from build123d import *

# Parameters (mm, degrees)
SKETCH_1_W                = 105
SKETCH_1_H                = 10
EXTRUDE_3_DEPTH           = 10
EXTRUDE_3_DEPTH_BACK      = 20
SKETCH_11_R               = 105
SKETCH_11_R_2             = 100
EXTRUDE_START             = 20
SKETCH_12_R               = 105
SKETCH_12_R_2             = 100
EXTRUDE_4_DEPTH           = 20
SKETCH_4_R                = 25.5
SKETCH_4_R_2              = 20.5
EXTRUDE_6_DEPTH           = 20
EXTRUDE_START_2           = -31.598350223
EXTRUDE_7_OUTLINE_R       = 26
EXTRUDE_7_OUTLINE_R_2     = 21
EXTRUDE_7_DEPTH           = 30.598350223
SKETCH_6_R                = 20
CUT_EXTRUDE_1_DEPTH       = 174.040821302
CUT_EXTRUDE_8_DEPTH       = 10
CUT_EXTRUDE_START         = -4.05
SKETCH_17_W               = 12.2
SKETCH_17_H               = 22.6
CUT_EXTRUDE_9_DEPTH       = 6.15
CUT_EXTRUDE_START_2       = -35
CUT_EXTRUDE_10_DEPTH      = 35.9
SKETCH_21_W               = 12.48598734
SKETCH_21_H               = 3.935393954
CUT_EXTRUDE_11_DEPTH      = 174.040821302
SKETCH_23_W               = 21.5
SKETCH_23_H               = 4
MIRROR_START              = -126.5
MIRROR_3_OUTLINE_R        = 26
MIRROR_3_OUTLINE_R_2      = 24
MIRROR_3_DEPTH            = 21.5
SKETCH_24_R               = 20
CUT_EXTRUDE_12_DEPTH      = 174.040821302
SKETCH_25_W               = 5.25
SKETCH_25_H               = 10
CUT_EXTRUDE_13_DEPTH      = 1
EXTRUDE_8_DEPTH           = 35
FILLET_1_R                = 10
FILLET_1_OF_MIRROR_4_R    = 10
M5X0_8_1_D                = 4.2
SKETCH_38_R               = 2.55
CUT_EXTRUDE_17_DEPTH      = 190.567335177
M5X0_8_2_D                = 4.2
CUT_EXTRUDE_18_DEPTH      = 183.219119633
CUT_EXTRUDE_18_DEPTH_BACK = 183.219119633
SKETCH_39_R               = 2.55
CUT_EXTRUDE_14_DEPTH      = 183.219119633
CUT_EXTRUDE_14_DEPTH_BACK = 183.219119633
SKETCH_34_W               = 208.658629851
SKETCH_34_H               = 276.195432186


with BuildPart() as part:
    # 草图1 → 旋转1 (revolve)
    with BuildSketch(Plane(origin=(0, 0, 0), x_dir=(1, 0, 0), z_dir=(0, 1, 0))):
        with Locations((52.5, 5)):
            Rectangle(SKETCH_1_W, SKETCH_1_H)
    revolve(axis=Axis((0, 0, 0), (0, 0, -1)))

    # 草图11 → 凸台-拉伸3 (add, two sides: drawn at the far end of the back side and taken through both)
    with BuildSketch(Plane.XY.offset(-EXTRUDE_3_DEPTH_BACK)):
        Circle(SKETCH_11_R)
        Circle(SKETCH_11_R_2, mode=Mode.SUBTRACT)
    extrude(amount=EXTRUDE_3_DEPTH + EXTRUDE_3_DEPTH_BACK)

    # 草图12 → 凸台-拉伸4 (add)
    with BuildSketch(Plane.XY.offset(10).offset(EXTRUDE_START)):
        Circle(SKETCH_12_R)
        Circle(SKETCH_12_R_2, mode=Mode.SUBTRACT)
    extrude_4 = extrude(amount=-EXTRUDE_4_DEPTH)

    # 镜向1: 凸台-拉伸4 across plane
    add(extrude_4.mirror(Plane.XY.offset(-5)))

    # 草图4 → 凸台-拉伸6 (add)
    with BuildSketch(Plane(origin=(100, 0, 0), x_dir=(0, 0, -1), z_dir=(1, 0, 0))):
        with Locations((5, 0)):
            Circle(SKETCH_4_R)
        with Locations((5, 0)):
            Circle(SKETCH_4_R_2, mode=Mode.SUBTRACT)
    extrude(amount=EXTRUDE_6_DEPTH)

    # 凸台-拉伸7: read off the stored shape, not the designer's step
    # 凸台-拉伸7 outline → 凸台-拉伸7 (add)
    with BuildSketch(Plane(origin=(-100, 0, 0), x_dir=(0, 0, -1), z_dir=(1, 0, 0)).offset(EXTRUDE_START_2)):
        with Locations((5, 0)):
            Circle(EXTRUDE_7_OUTLINE_R)
        with Locations((5, 0)):
            Circle(EXTRUDE_7_OUTLINE_R_2, mode=Mode.SUBTRACT)
    extrude(amount=EXTRUDE_7_DEPTH)

    # 草图6 → 切除-拉伸1 (cut, through all)
    with BuildSketch(Plane.XY):
        with Locations((0, -70)):
            Circle(SKETCH_6_R)
        with Locations(Location((0, 70, 0), (0, 0, 180))):
            Circle(SKETCH_6_R)
    extrude(amount=-CUT_EXTRUDE_1_DEPTH, mode=Mode.SUBTRACT)

    # 草图16 → 切除-拉伸8 (cut)
    with BuildSketch(Plane(origin=(105, 0, 0), x_dir=(0, 0, -1), z_dir=(1, 0, 0))):
        with BuildLine():
            ThreePointArc((7.301532566, -5.323809524), (5, 5.8), (2.698467434, -5.323809524))
            ThreePointArc((2.698467434, -5.323809524), (5, -8.8), (7.301532566, -5.323809524))
        make_face()
    cut_extrude_8 = extrude(amount=-CUT_EXTRUDE_8_DEPTH, mode=Mode.SUBTRACT)

    # 草图17 → 切除-拉伸9 (cut)
    with BuildSketch(Plane(origin=(100, 0, 0), x_dir=(0, 0, -1), z_dir=(1, 0, 0)).offset(CUT_EXTRUDE_START)):
        with Locations((4.890474786, -5.5)):
            Rectangle(SKETCH_17_W, SKETCH_17_H)
    cut_extrude_9 = extrude(amount=CUT_EXTRUDE_9_DEPTH, mode=Mode.SUBTRACT)

    # 草图19 → 切除-拉伸10 (cut)
    with BuildSketch(Plane(origin=(95.95, 0, 0), x_dir=(0, 0, -1), z_dir=(1, 0, 0)).offset(CUT_EXTRUDE_START_2)):
        Polygon((-1.122566441, -16.8), (-1.122566441, 5.8), (-1.122566441, 10.8), (11.077433559, 10.8), (11.077433559, 5.8), (11.077433559, -16.8), (11.077433559, -21.6), (-1.122566441, -21.6), align=None)
    cut_extrude_10 = extrude(amount=CUT_EXTRUDE_10_DEPTH, mode=Mode.SUBTRACT)

    # 镜向2: 切除-拉伸8, 切除-拉伸9, 切除-拉伸10 across plane
    add(cut_extrude_8.mirror(Plane(origin=(0, 0, 0), x_dir=(0, 0, 1), z_dir=(1, 0, 0))), mode=Mode.SUBTRACT)
    add(cut_extrude_9.mirror(Plane(origin=(0, 0, 0), x_dir=(0, 0, 1), z_dir=(1, 0, 0))), mode=Mode.SUBTRACT)
    add(cut_extrude_10.mirror(Plane(origin=(0, 0, 0), x_dir=(0, 0, 1), z_dir=(1, 0, 0))), mode=Mode.SUBTRACT)

    # 草图21 → 切除-拉伸11 (cut, through all)
    with BuildSketch(Plane.XY):
        with Locations((-80.471231892, 15.58208287)):
            Rectangle(SKETCH_21_W, SKETCH_21_H)
        with Locations((-80.471231892, -26.38208287)):
            Rectangle(SKETCH_21_W, SKETCH_21_H)
        with Locations((80.471231892, -26.38208287)):
            Rectangle(SKETCH_21_W, SKETCH_21_H)
        with Locations((80.471231892, 15.58208287)):
            Rectangle(SKETCH_21_W, SKETCH_21_H)
    extrude(amount=-CUT_EXTRUDE_11_DEPTH, mode=Mode.SUBTRACT)

    # 草图23 → 切除-旋转1 (revolve, cut)
    with BuildSketch(Plane.XY.offset(-5), mode=Mode.PRIVATE) as cut_revolve_1_sk:
        with Locations((115.75, 26)):
            Rectangle(SKETCH_23_W, SKETCH_23_H)
    revolve(cut_revolve_1_sk.sketch.rotate(Axis((120, 0, -5), (-1, 0, 0)), 90), axis=Axis((120, 0, -5), (-1, 0, 0)), mode=Mode.SUBTRACT)

    # 镜向3: read off the stored shape, not the designer's step
    # 镜向3 outline → 镜向3 (cut)
    with BuildSketch(Plane.YZ.offset(MIRROR_START)):
        with Locations((0, -5)):
            Circle(MIRROR_3_OUTLINE_R)
        with Locations((0, -5)):
            Circle(MIRROR_3_OUTLINE_R_2, mode=Mode.SUBTRACT)
    extrude(amount=MIRROR_3_DEPTH, mode=Mode.SUBTRACT)

    # 草图24 → 切除-拉伸12 (cut, through all)
    with BuildSketch(Plane.XY):
        Circle(SKETCH_24_R)
        with BuildLine():
            Line((-86.979425588, 23.120975852), (-48.321903105, 12.844986584))
            ThreePointArc((-48.321903105, 12.844986584), (0, 50), (48.321903105, 12.844986584))
            Line((48.321903105, 12.844986584), (86.979425588, 23.120975852))
            ThreePointArc((86.979425588, 23.120975852), (0, 90), (-86.979425588, 23.120975852))
        make_face()
        with BuildLine():
            Line((46.279615655, -18.926097718), (83.303308179, -34.066975893))
            ThreePointArc((83.303308179, -34.066975893), (0, -90), (-83.303308179, -34.066975893))
            Line((-83.303308179, -34.066975893), (-46.279615655, -18.926097718))
            ThreePointArc((-46.279615655, -18.926097718), (0, -50), (46.279615655, -18.926097718))
        make_face()
    extrude(amount=-CUT_EXTRUDE_12_DEPTH, mode=Mode.SUBTRACT)

    # 草图25 → 切除-拉伸13 (cut)
    with BuildSketch(Plane.XZ.offset(-5.8)):
        with Locations((99.475, -5)):
            Rectangle(SKETCH_25_W, SKETCH_25_H)
    extrude(amount=-CUT_EXTRUDE_13_DEPTH, mode=Mode.SUBTRACT)

    # 草图26 → 凸台-拉伸8 (add, symmetric)
    with BuildSketch(Plane.XY.offset(-5)):
        with BuildLine():
            Line((-10, 104.522724802), (-10, 119.522724802))
            Line((-10, 119.522724802), (10, 119.522724802))
            Line((10, 119.522724802), (10, 104.522724802))
            ThreePointArc((10, 104.522724802), (0, 105), (-10, 104.522724802))
        make_face()
    extrude_8 = extrude(amount=EXTRUDE_8_DEPTH, both=True)

    # 圆角1
    fillet_1_edges = [part.edges().sort_by_distance(p)[0] for p in [
        (0, 119.522724802, -40),
        (0, 119.522724802, 30),
    ]]
    fillet(fillet_1_edges, radius=FILLET_1_R)

    # 镜向4: 凸台-拉伸8 across plane
    add(extrude_8.mirror(Plane.ZX))

    # 圆角1 of 镜向4
    fillet_1_of_mirror_4_edges = [part.edges().sort_by_distance(p)[0] for p in [
        (0, -119.522724802, -40),
        (0, -119.522724802, 30),
    ]]
    fillet(fillet_1_of_mirror_4_edges, radius=FILLET_1_OF_MIRROR_4_R)

    # M5x0.8 螺纹孔1 (through all)
    with Locations(Plane(origin=(10, 0, 0), x_dir=(0, 0, -1), z_dir=(1, 0, 0))):
        with Locations((-12.5, 111.675356556), (5, 111.675356556), (22.5, 111.675356556)):
            m5x0_8_1 = Hole(M5X0_8_1_D / 2)

    # 草图38 → 切除-拉伸17 (cut, through all)
    with BuildSketch(Plane(origin=(10, 0, 0), x_dir=(0, 0, -1), z_dir=(1, 0, 0))):
        with Locations((-12.5, 111.675356556)):
            Circle(SKETCH_38_R)
        with Locations((5, 111.675356556)):
            Circle(SKETCH_38_R)
        with Locations((22.5, 111.675356556)):
            Circle(SKETCH_38_R)
    cut_extrude_17 = extrude(amount=-CUT_EXTRUDE_17_DEPTH, mode=Mode.SUBTRACT)

    # 镜向5: M5x0.8 螺纹孔1, 切除-拉伸17 across plane
    add(m5x0_8_1.mirror(Plane.ZX), mode=Mode.SUBTRACT)
    add(cut_extrude_17.mirror(Plane.ZX), mode=Mode.SUBTRACT)

    # M5x0.8 螺纹孔2 (through all)
    with Locations(Plane.XY):
        with Locations((-35, 0), (35, 0)):
            Hole(M5X0_8_2_D / 2)

    # 草图39 → 切除-拉伸18 (cut, two sides: drawn at the far end of the back side and taken through both)
    with BuildSketch(Plane.XY.offset(-CUT_EXTRUDE_18_DEPTH_BACK)):
        with Locations((-35, 0)):
            Circle(SKETCH_39_R)
        with Locations((35, 0)):
            Circle(SKETCH_39_R)
    extrude(amount=CUT_EXTRUDE_18_DEPTH + CUT_EXTRUDE_18_DEPTH_BACK, mode=Mode.SUBTRACT)

    # 草图34 → 切除-拉伸14 (cut, two sides: drawn at the far end of the back side and taken through both)
    with BuildSketch(Plane.XY.offset(-CUT_EXTRUDE_14_DEPTH_BACK)):
        with Locations((104.829314926, -9.366190691)):
            Rectangle(SKETCH_34_W, SKETCH_34_H)
    extrude(amount=CUT_EXTRUDE_14_DEPTH + CUT_EXTRUDE_14_DEPTH_BACK, mode=Mode.SUBTRACT)


solid = part.part
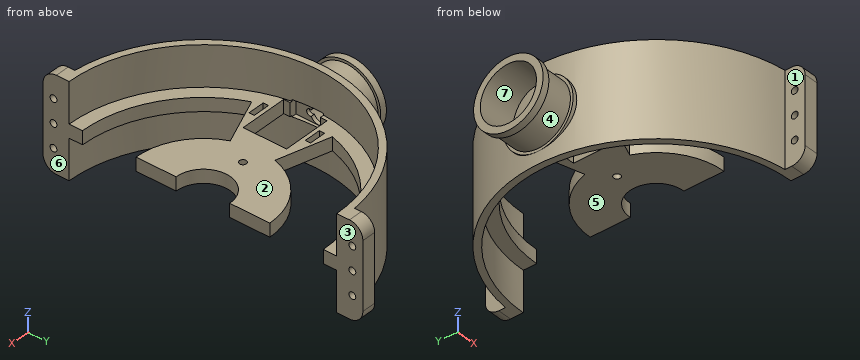
Part model, mm, in its own coordinate system. Face numbers are marked on the shaded views. A direction names the side the tool comes from. Round coordinates to 2 decimals unless told otherwise and drop trailing zeros. Loops run counter-clockwise (first coordinate to the right, second up) from the corner with the lowest first, then second, coordinate; pieces in that order, holes last. Notation, with made-up numbers: (17, -21) - (71, -21) arc R29 cw to (71, 4) - close; hole circle Ø11 at (9.5, 45.5). An arc over 180 degrees is marked (long way). Answer as a JSON object with one key per item and string values.
Item 1: Band-saw the part on C-C on y = -97. List the corners of the cut face in (x, z).
Output:
{"outline": "(-40.2, -40) - (-24.31, -40) - (-24.31, -10) - (0.5, -10) - (0.5, 0) - (-24.31, 0) - (-24.31, 30) - (-40.2, 30) - close"}
Item 2: Tool access for the marked faces 1, 2 and 3: list every direction of +Z, -Z, +X, -X, +Y, -Y with a clear straight run to the whole face (end or side of a thin tool).
Output:
{"face 1": "+Z, -Z, -X, -Y", "face 2": "+Z, +X", "face 3": "+Z, -Z, +X, +Y, -Y"}
Item 3: Wall check: L1, parallel to Y at x = -5.5, z = -22.5; L2, parallel to Y at x = -5, z = -5; L3, parallel to Z at x = -32.5, y = 92. Give the ranges that are in metal, low to high.
Output:
{"L1": "-119.52 to -114.23, -109.13 to -99.85, 99.85 to 109.13, 114.23 to 119.52", "L2": "-119.52 to -114.23, -109.13 to -89.86, -49.75 to -19.36, 19.36 to 49.75, 89.86 to 109.13, 114.23 to 119.52", "L3": "-10 to 0"}
Item 4: Band-saw the part on A-A on x = -93. List the corners of the cut face in (y, z).
Output:
{"outline": "(-48.74, -40) - (-36.76, -40) - (-36.76, -10) - (-21.6, -10) - (-21.6, 0) - (-36.76, 0) - (-36.76, 30) - (-48.74, 30) - close; (10.8, -10) - (36.76, -10) - (36.76, -40) - (48.74, -40) - (48.74, 30) - (36.76, 30) - (36.76, 0) - (10.8, 0) - close"}
Item 5: Band-saw the part on D-D on x = -27. List the corners of the cut face in (y, z).
Output:
{"outline": "(-101.47, -40) - (-96.29, -40) - (-96.29, -10) - (-85.85, -10) - (-85.85, 0) - (-96.29, 0) - (-96.29, 30) - (-101.47, 30) - close; (-42.08, -10) - (42.08, -10) - (42.08, 0) - (-42.08, 0) - close; (85.85, -10) - (96.29, -10) - (96.29, -40) - (101.47, -40) - (101.47, 30) - (96.29, 30) - (96.29, 0) - (85.85, 0) - close"}
Item 6: Pull direction Z, two halves, no side cores. Call the marked faces 4, 5, 6 and 7: pulls with the +Z half, pulls with the -Z half, needs draft (parallel to the pull), parting line crosses it, or undercut.
Output:
{"face 4": "parting line crosses it", "face 5": "pulls with the -Z half", "face 6": "needs draft", "face 7": "undercut"}
Item 7: Band-saw the part on B-B on z = 12.5. State how many separate pieces and enclosed holes the cut face has, plus the area to 3 significant figures.
Output:
{"separate pieces": "3", "enclosed holes": "0", "area": "2,120 mm2"}
Item 8: Pin check, flat tips, straight feed: pin 1 (4 mm diameter, centred on x = -93.5, z = 1.5, fed in from -Y); pin 2 (4.5 mm diameter, centred on y = 16, z = -6.5, fed in from +X); pin 3 (10 mm diameter, centred on x = -24.5, z = -26, fed in from -Y). Stop position of each tip, or through.
Output:
{"pin 1": "y = -51.5", "pin 2": "x = -8.18", "pin 3": "y = -103.17"}
